Input: part model. Units: mm. Frame: model coordinates. A direction names the side the tool comes from. Round coordinates to 2 decimals unless told otherwise and drop trailing zeros. Order: outer loops, then holes, each group sorted by start corner. A loop starts at its lowest first (then second) coordinate and runs counter-clockwise, first axis right, second up.
Item 1: Mould query, pull axis Y, two halves, no side actions, for faces 5 (the flat face through (28.564, 26.856, 9.951)), 6 (the flat face through (26, 3, -10)), 7 (the cylindrical face through (0.603, 1.479, 11.605)), 8 (the flat face through (20, 16.75, -9)). Classes: released by +Y, released by -Y, zero draft, split by the parting line, or undercut.
Item 2: Line query: L1, parallel to Y at x = 16, z = -19.5; L2, parallel to Y at x = 18, z = 19; L3, parallel to X at y = 38.5, z = -9. Output: solid intervals per line, ascending.
Item 3: Cut plane C-C on z = -19.5. Output: boundary loops of the cut face in (x, y).
Item 4: Cut plane A-A on y = 12.5. Output: boundary loops of the cut face in (x, z), then the cut area to 3 significant figures.
Item 5: First-contact query: pin 1 (1.5 mm diameter, centred on x = -16.5, y = 8.5, fed in from +Z); pin 2 (2.5 mm diameter, centred on x = 10.15, z = 0, fed in from +Y); pin 3 (3 mm diameter, centred on y = 7.5, z = -5.5, fed in from -X); pin 4 (10 mm diameter, centred on x = -22, z = 1.5, fed in from +Y). Flat tips, straight axial feed; report the tip coordinate or a pass-through.
Item 6: Cut plane B-B on x = -10.15. Output: boundary loops of the cut face in (y, z) (3 decimals), then the cut area to 3 significant figures.
Item 7: Reachability of faces 1 (the flat face through (-3, 3, 7)), 2 (the flat face through (-37.038, 26.856, -6.273)), 3 (the flat face through (-30.44, 14.39, 12.75)), 4 (the flat face through (-20.72, 26.86, 31.34)) from +Z, -Z, +X, -X, +Y, -Y: full face, straight path, thin tool, end or side. Return the list, or none.
```python
from build123d import *

# Parameters (mm, degrees)
SKETCH1_R           = 0.5
SKETCH1_R_2         = 1.575
BOSS_EXTRUDE1_DEPTH = 3
BOSS_EXTRUDE2_START = 30
SKETCH2_W           = 60
SKETCH2_H           = 40
SKETCH2_R           = 1.689490446
SKETCH2_W_2         = 41
SKETCH2_H_2         = 20.5
BOSS_EXTRUDE2_DEPTH = 3
BOSS_EXTRUDE3_START = -23.72
SKETCH2_2_W         = 60
SKETCH2_2_H         = 40
SKETCH2_2_R         = 1.689490446
SKETCH2_2_W_2       = 41
SKETCH2_2_H_2       = 20.5
BOSS_EXTRUDE3_DEPTH = 3
CUT_EXTRUDE1_DEPTH  = 10


with BuildPart() as part:
    # Sketch1 → Boss-Extrude1 (new body)
    with BuildSketch(Plane(origin=(0, 0, 0), x_dir=(1, 0, 0), z_dir=(0, 1, 0))):
        with BuildLine():
            Line((33.702537367, -18.076984677), (32.005152982, -14.165810341))
            ThreePointArc((32.005152982, -14.165810341), (32.106828614, 13.933827771), (11.51335986, 33.052118612))
            Line((11.51335986, 33.052118612), (9.815975474, 36.963292947))
            Line((9.815975474, 36.963292947), (7.063961593, 35.768964852))
            Line((7.063961593, 35.768964852), (7.77744177, 34.124938088))
            ThreePointArc((7.77744177, 34.124938088), (-19.979563219, 28.73703279), (-34.697157454, 4.594264319))
            Line((-34.697157454, 4.594264319), (-39.463419759, 15.576857865))
            Line((-39.463419759, 15.576857865), (-42.291947314, 14.577141972))
            Line((-42.291947314, 14.577141972), (-34.916382331, -2.417900937))
            ThreePointArc((-34.916382331, -2.417900937), (-32.106828614, -13.933827771), (-25.614551861, -23.85151427))
            Line((-25.614551861, -23.85151427), (-18.322186149, -40.654846416))
            Line((-18.322186149, -40.654846416), (-15.576857865, -39.463419759))
            Line((-15.576857865, -39.463419759), (-20.34312017, -28.480826213))
            ThreePointArc((-20.34312017, -28.480826213), (7.343177958, -34.221013098), (30.237043308, -17.627286007))
            Line((30.237043308, -17.627286007), (30.950523486, -19.271312771))
            Line((30.950523486, -19.271312771), (33.702537367, -18.076984677))
        make_face()
        with Locations(Location((0, -16.15, 0), (0, 0, 270))):
            Circle(SKETCH1_R, mode=Mode.SUBTRACT)
        with BuildLine():
            ThreePointArc((0, -12.65), (0.5, -13.15), (0, -13.65))
            ThreePointArc((0, -13.65), (-0.5, -13.15), (0, -12.65))
        make_face(mode=Mode.SUBTRACT)
        with BuildLine():
            ThreePointArc((0, -8.575), (1.575, -10.15), (0, -11.725))
            ThreePointArc((0, -11.725), (-1.575, -10.15), (0, -8.575))
        make_face(mode=Mode.SUBTRACT)
        with BuildLine():
            ThreePointArc((0, -6.005210608), (0.5, -6.505210608), (0, -7.005210608))
            ThreePointArc((0, -7.005210608), (-0.5, -6.505210608), (0, -6.005210608))
        make_face(mode=Mode.SUBTRACT)
        with BuildLine():
            ThreePointArc((11.725, 0), (10.15, -1.575), (8.575, 0))
            ThreePointArc((8.575, 0), (10.15, 1.575), (11.725, 0))
        make_face(mode=Mode.SUBTRACT)
        with Locations(Location((-16.15, 0, 0), (0, 0, 270))):
            Circle(SKETCH1_R, mode=Mode.SUBTRACT)
        with BuildLine():
            ThreePointArc((-12.65, 0), (-13.15, -0.5), (-13.65, 0))
            ThreePointArc((-13.65, 0), (-13.15, 0.5), (-12.65, 0))
        make_face(mode=Mode.SUBTRACT)
        with Locations(Location((-10.15, 0, 0), (0, 0, 270))):
            Circle(SKETCH1_R_2, mode=Mode.SUBTRACT)
        with Locations(Location((-6.505210608, 0, 0), (0, 0, 270))):
            Circle(SKETCH1_R, mode=Mode.SUBTRACT)
        with BuildLine():
            ThreePointArc((4.401273885, 0), (3.11217061, -3.11217061), (0, -4.401273885))
            ThreePointArc((0, -4.401273885), (-4.401273885, 0), (0, 4.401273885))
            Line((0, 4.401273885), (0, 0))
            Line((0, 0), (4.037455609, 1.752188351))
            ThreePointArc((4.037455609, 1.752188351), (4.309359567, 0.894780386), (4.401273885, 0))
        make_face(mode=Mode.SUBTRACT)
        with BuildLine():
            ThreePointArc((7.005210608, 0), (6.505210608, -0.5), (6.005210608, 0))
            ThreePointArc((6.005210608, 0), (6.505210608, 0.5), (7.005210608, 0))
        make_face(mode=Mode.SUBTRACT)
        with BuildLine():
            ThreePointArc((0, 7.005210608), (0.5, 6.505210608), (0, 6.005210608))
            ThreePointArc((0, 6.005210608), (-0.5, 6.505210608), (0, 7.005210608))
        make_face(mode=Mode.SUBTRACT)
        with BuildLine():
            ThreePointArc((13.65, 0), (13.15, -0.5), (12.65, 0))
            ThreePointArc((12.65, 0), (13.15, 0.5), (13.65, 0))
        make_face(mode=Mode.SUBTRACT)
        with Locations(Location((16.15, 0, 0), (0, 0, 270))):
            Circle(SKETCH1_R, mode=Mode.SUBTRACT)
        with BuildLine():
            ThreePointArc((0, 11.725), (1.575, 10.15), (0, 8.575))
            ThreePointArc((0, 8.575), (-1.575, 10.15), (0, 11.725))
        make_face(mode=Mode.SUBTRACT)
        with BuildLine():
            ThreePointArc((0, 13.65), (0.5, 13.15), (0, 12.65))
            ThreePointArc((0, 12.65), (-0.5, 13.15), (0, 13.65))
        make_face(mode=Mode.SUBTRACT)
        with Locations(Location((0, 16.15, 0), (0, 0, 270))):
            Circle(SKETCH1_R, mode=Mode.SUBTRACT)
    extrude(amount=BOSS_EXTRUDE1_DEPTH)

    # Sketch2 → Boss-Extrude2 (add)
    with BuildSketch(Plane(origin=(0, 0, 0), x_dir=(0.3981093648941227, 0, 0.9173379603960573), z_dir=(-0.9173379603960573, 0, 0.3981093648941227)).offset(BOSS_EXTRUDE2_START)):
        with Locations((0, 23)):
            Rectangle(SKETCH2_W, SKETCH2_H)
        with Locations(Location((-23.689490446, 31.9, 0), (0, 0, 180))):
            Circle(SKETCH2_R, mode=Mode.SUBTRACT)
        with Locations(Location((-23.689490446, 22.1, 0), (0, 0, 180))):
            Circle(SKETCH2_R, mode=Mode.SUBTRACT)
        with Locations(Location((23.689490446, 22.1, 0), (0, 0, 180))):
            Circle(SKETCH2_R, mode=Mode.SUBTRACT)
        with Locations(Location((23.689490446, 31.9, 0), (0, 0, 180))):
            Circle(SKETCH2_R, mode=Mode.SUBTRACT)
        with Locations((0, 27)):
            Rectangle(SKETCH2_W_2, SKETCH2_H_2, mode=Mode.SUBTRACT)
    extrude(amount=BOSS_EXTRUDE2_DEPTH)

    # Sketch2<2> → Boss-Extrude3 (add)
    with BuildSketch(Plane(origin=(0, 0, 0), x_dir=(0.3981093648941227, 0, 0.9173379603960573), z_dir=(-0.9173379603960573, 0, 0.3981093648941227)).offset(BOSS_EXTRUDE3_START)):
        with Locations((0, 23)):
            Rectangle(SKETCH2_2_W, SKETCH2_2_H)
        with Locations(Location((-23.689490446, 31.9, 0), (0, 0, 180))):
            Circle(SKETCH2_2_R, mode=Mode.SUBTRACT)
        with Locations(Location((-23.689490446, 22.1, 0), (0, 0, 180))):
            Circle(SKETCH2_2_R, mode=Mode.SUBTRACT)
        with Locations(Location((23.689490446, 22.1, 0), (0, 0, 180))):
            Circle(SKETCH2_2_R, mode=Mode.SUBTRACT)
        with Locations(Location((23.689490446, 31.9, 0), (0, 0, 180))):
            Circle(SKETCH2_2_R, mode=Mode.SUBTRACT)
        with Locations((0, 27)):
            Rectangle(SKETCH2_2_W_2, SKETCH2_2_H_2, mode=Mode.SUBTRACT)
    extrude(amount=BOSS_EXTRUDE3_DEPTH)

    # Sketch1<3> → Cut-Extrude1 (cut)
    with BuildSketch(Plane(origin=(0, 0, 0), x_dir=(1, 0, 0), z_dir=(0, 1, 0))):
        with BuildLine():
            Line((0, 1.313954222), (0, 0))
            Line((0, 0), (4.037455609, 1.752188351))
            ThreePointArc((4.037455609, 1.752188351), (2.414472094, 3.679882651), (0, 4.401273885))
            Line((0, 4.401273885), (0, 1.313954222))
        make_face()
    extrude(amount=CUT_EXTRUDE1_DEPTH, mode=Mode.SUBTRACT)


solid = part.part
```
From the geometry:
1. face 5: undercut
1. face 6: released by +Y
1. face 7: zero draft
1. face 8: undercut
2. L1: y = 0 to 16.75, 37.25 to 43
2. L2: y = 0 to 3
2. L3: x = -39.88 to -36.61, 18.68 to 21.95
3. outline: (-29.06, 0) - (29.06, 0) - (29.06, 3) - (17.39, 3) - (17.39, 16.75) - (14.12, 16.75) - (14.12, 3) - (-29.06, 3) - close; (14.12, 37.25) - (17.39, 37.25) - (17.39, 43) - (14.12, 43) - close
4. outline: (-42.22, -14.38) - (-39.46, -15.58) - (-15.58, 39.46) - (-18.33, 40.66) - close; (7.06, -35.77) - (9.82, -36.96) - (33.7, 18.08) - (30.95, 19.27) - close
4. area: 360 mm2
5. pin 1: stops at z = 40.19
5. pin 2: passes through
5. pin 3: stops at x = -39.01
5. pin 4: stops at y = 3
6. outline: (0, -33.496) - (3, -33.496) - (3, -1.575) - (0, -1.575) - close; (0, 1.575) - (3, 1.575) - (3, 33.496) - (0, 33.496) - close
6. area: 192 mm2
7. face 1: +Y
7. face 2: +Z, +X
7. face 3: +Z, -X, +Y
7. face 4: -Z, -X
